```python
from build123d import *

# Parameters (mm, degrees)
F0_W     = 270.8007246256
F0_H     = 385.7633024454
F1_DEPTH = 82.55
F3_DEPTH = 508
F5_R     = 8.6846383289
F5_R_2   = 24.5957658021
F6_DEPTH = 381
F7_DEPTH = 1016


with BuildPart() as f1:
    # F0 (on Top) → F1 (new body)
    with BuildSketch(Plane.XY):
        with Locations((12.6297399402, 24.1259709001)):
            Rectangle(F0_W, F0_H)
    extrude(amount=F1_DEPTH)

    # F2 (on face) → F3 (cut)
    with BuildSketch(Plane.YZ.offset(148.030102253)):
        Polygon((217.0076221228, 82.55), (-168.7556803226, 82.55), (217.0076221228, 0), align=None)
    extrude(amount=-F3_DEPTH, mode=Mode.SUBTRACT)

    # F5 (on face) → F6 (cut)
    with BuildSketch(Plane(origin=(-122.7706223726, 0, 0), x_dir=(0, -1, 0), z_dir=(-1, 0, 0))):
        with Locations((-82.6604217291, 12.0333293453)):
            Circle(F5_R)
        with Locations((111.8754446507, 26.6235191375)):
            Circle(F5_R_2)
    extrude(amount=-F6_DEPTH, mode=Mode.SUBTRACT)

    # F4 (on face) → F7 (cut)
    with BuildSketch(Plane(origin=(0, 9.5021501125, 44.4043707783), x_dir=(1, 0, 0), z_dir=(0, 0.2092538463, 0.9778613541))):
        Polygon((148.030102253, 212.2033672174), (12.6297399402, 212.2033672174), (148.030102253, -182.2935630794), align=None)
        Polygon((-122.7706223726, -182.2935630794), (12.6297399402, 212.2033672174), (-122.7706223726, 212.2033672174), align=None)
    extrude(amount=-F7_DEPTH, mode=Mode.SUBTRACT)


solid = f1.part
```
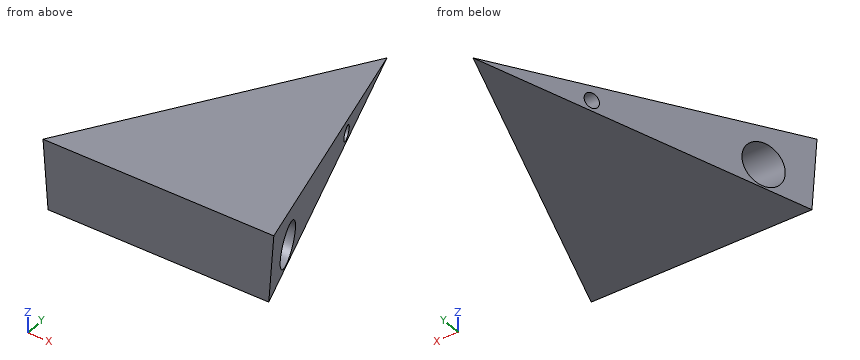
For this review, take the finished solid that the model builds, in its own axes (mm). Round coordinates to 2 decimals unless told otherwise and drop trailing zeros. Write each loop counter-clockwise with the first axis right and the second up, starting at its lowest first coordinate (ties: lowest second). Pieces come first, ordered by that corner, then holes. Notation, with made-up numbers: (57.25, 30.5) -> (89.25, 30.5) arc R8 ccw to (89.25, 41.5) -> close; hole circle Ø8 at (46.25, 49.25). An arc over 180 degrees is marked (long way). One line per question, with ' | ' between items. Start each with the question number.
(1) Add section B-B, the plane z = 36. Write out the cut boundary in (x, y), plus the area to 3 significant figures.
(2) Insertion check: P1, Ø20, axis at y = 82.66, z = 12.03, coming from the +X side; P2, Ø5, axis at x = 42.5, y = 32, coming from the +Z side (3 decimals); P3, Ø3, axis at x = 14.5, y = 115, coming from the +Z side; P4, Ø6, axis at y = -78.5, z = 68.5, coming from the -X side. Each pin has a flat end and moves straight along its axis. Give the tip position at first contact, or say it passes through.
(3) Add section D-D, the plane x = 31. Write out the cut boundary in (y, z), plus the area to 3 significant figures.
(4) Add section C-C, the plane x = -70.5. Write out the cut boundary in (y, z).
(5) For line 1 along Z through (x, y) = (79.5, -120); line 2 along Z through (x, y) = (42, 75.5); line 3 along X through (y, z) = (-133, 42), list the stretches that pass through material, from the lowest coordinate up. Write a range as from..to.
(6) Add section A-A, the plane y = -131. Write out the cut boundary in (x, z).
Answer list:
1) outline: (-119.43, -168.76) -> (144.69, -168.76) -> (133.23, -134.61) -> (-107.97, -134.61) -> close; (-92.71, -89.14) -> (117.96, -89.14) -> (71.68, 48.78) -> (-46.42, 48.78) -> close | area: 31,300 mm²
2) P1: x = 62.02 | P2: z = 40.125 | P3: z = 22.15 | P4: through
3) outline: (-168.76, 0) -> (162.27, 0) -> (164.67, 11.2) -> (-168.76, 82.55) -> close; hole circle Ø49.19 at (-111.88, 26.62); hole circle Ø17.37 at (82.66, 12.03) | area: 13,500 mm²
4) outline: (-168.76, 0) -> (-30.68, 0) -> (-19.83, 50.68) -> (-168.76, 82.55) -> close; hole circle Ø49.19 at (-111.88, 26.62)
5) line 1: 0..3.41, 49.84..72.12 | line 2: 0..7.12, 16.95..30.28 | line 3: -107.86..133.12
6) outline: (-109.52, 74.47) -> (-107.19, 42.09) -> (132.45, 42.09) -> (134.78, 74.47) -> close; (-104.97, 11.16) -> (-104.17, 0) -> (129.43, 0) -> (130.23, 11.16) -> close
